Geometry: see drawing. Coordinates: mm, zero at the bounding-box minimum. A direction names the side the tool comes from. Coordinates: 2 decimals unless noted, no trailing zeros. Write each loop counter-clockwise with the first axis right and the second up, starting at its lowest first coordinate (ties: lowest second). Pieces come first, ordered by that corner, then holes. Notation, with made-up numbers: (-12, -38.75) - (5, -38.75) arc R6 cw to (5, -31.75) - close; hole circle Ø7 at (-8.75, 33). An arc over 180 degrees is marked (long way). Use a Markdown table: item, result. Add a question column.
Q1. Section query B-B (z = 306). Return the cut outline in (x, y), then the cut area to 3 significant figures.
Q2. Section query C-C (x = 110.5). Return the cut outline in (y, z).
Q3. Material intervals for probe 1 along X at (y, z) = (33.5, 262); probe 2 along Z at (x, y) = (48, 44); probe 3 along Z at (x, y) = (138, 27), sorted ascending. Write a range as from..to.
Q4. Pin query (flat end, axial travel): P1, Ø10, axis at x = 90, y = 11, coming from the -Z side; P2, Ø6, axis at y = 31, z = 49, coming from the -X side. Return the tip coordinate at first contact, or that it passes through.
Q5. Section query A-A (y = 39). Return the cut outline in (x, z), then the cut area to 3 significant figures.
Q6. Set-up query: the marked faces 1 and 2. Return all of +Z, -Z, +X, -X, +Y, -Y with unobstructed straight access to the full face (end or side cutting, diameter ignored); none if empty.
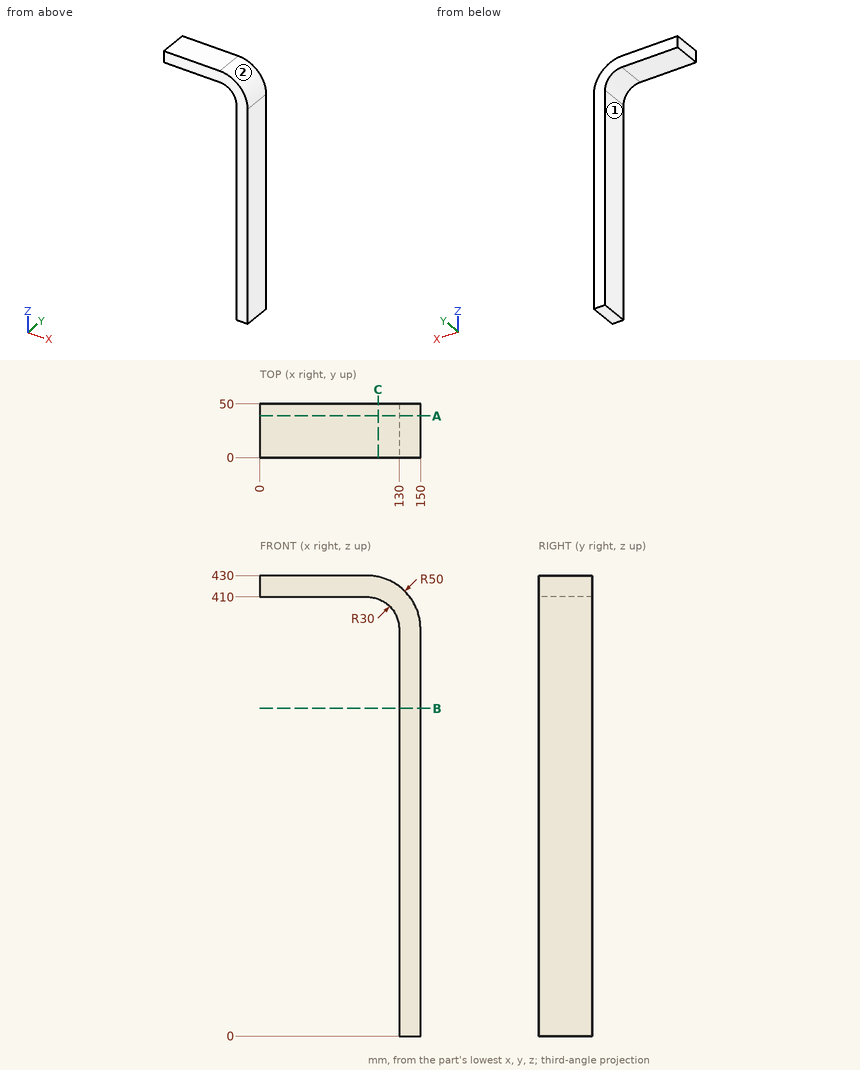
Values follow:
| question | item | result |
|---|---|---|
| 1 | outline | (130, 0) - (150, 0) - (150, 50) - (130, 50) - close |
| 1 | area | 1,000 mm2 |
| 2 | outline | (0, 408.1) - (50, 408.1) - (50, 428.89) - (0, 428.89) - close |
| 3 | probe 1 | 130..150 |
| 3 | probe 2 | 410..430 |
| 3 | probe 3 | 0..412.5 |
| 4 | P1 | z = 410 |
| 4 | P2 | x = 130 |
| 5 | outline | (0, 410) - (100, 410) arc R30 cw to (130, 380) - (130, 0) - (150, 0) - (150, 380) arc R50 ccw to (100, 430) - (0, 430) - close |
| 5 | area | 10,900 mm2 |
| 6 | face 1 | -Z, -X, +Y, -Y |
| 6 | face 2 | +Z, +X, +Y, -Y |
